```python
from build123d import *

# Parameters (mm, degrees)
F0_W     = 4.2418
F0_H     = 20.1168
F7_DEPTH = 17.78
F1_R     = 2.130855
F2_DEPTH = 7.62
F1_R_2   = 10.202132
F3_DEPTH = 1.27


with BuildPart() as f7:
    # F0 (on Top) → F7 (new body)
    with BuildSketch(Plane.XY):
        Rectangle(F0_W, F0_H)
    extrude(amount=F7_DEPTH)

    # F1 (on offset) → F2 (join)
    with BuildSketch(Plane.XY.offset(17.78)):
        Circle(F1_R)
    extrude(amount=F2_DEPTH)

    # F1 (on offset) → F3 (join)
    with BuildSketch(Plane.XY.offset(17.78)):
        Circle(F1_R_2)
        Circle(F1_R, mode=Mode.SUBTRACT)
    extrude(amount=F3_DEPTH)


solid = f7.part
```
Input: part model. Units: mm. Frame: model coordinates. A direction names the side the tool comes from. Give positions to 0.01 mm unless a question says otherwise; leave off trailing zeros. Loops run counter-clockwise (first coordinate to the right, second up) from the corner with the lowest first, then second, coordinate; pieces in that order, holes last.
1) Section query A-A on x = 0. Return the cut outline in (y, z).
A:
outline: (-10.2, 17.78) - (-10.06, 17.78) - (-10.06, 0) - (10.06, 0) - (10.06, 17.78) - (10.2, 17.78) - (10.2, 19.05) - (2.13, 19.05) - (2.13, 25.4) - (-2.13, 25.4) - (-2.13, 19.05) - (-10.2, 19.05) - close
2) Section query D-D on y = -6. Return the cut outline in (x, z).
A:
outline: (-8.25, 17.78) - (-2.12, 17.78) - (-2.12, 0) - (2.12, 0) - (2.12, 17.78) - (8.25, 17.78) - (8.25, 19.05) - (-8.25, 19.05) - close
3) Reachability of faces 1 (the cylindrical face through (-0.46, -2.08, 22.18)), 2 (the flat face through (2.121, 0, 9)), 3 (the flat face through (-2.121, 0, 9)) from +Z, -Z, +X, -X, +Y, -Y: full face, straight path, thin tool, end or side. Return the list, or none.
A:
face 1: +Z
face 2: -Z, +X, +Y, -Y
face 3: -Z, -X, +Y, -Y
4) Section query C-C on z = 18.5. Return the cut outline in (x, y), and give its area (3 significant figures).
A:
outline: circle Ø20.4 at (0, 0)
area: 327 mm2
5) Line query: L1, parallel to Z at x = 1.75, y = 1.5; L2, parallel to X at y = 7.5, z = 16; L3, parallel to Z at x = -8.75, y = -3. Output: solid intervals per line, ascending.
A:
L1: z = 0 to 19.05
L2: x = -2.12 to 2.12
L3: z = 17.78 to 19.05
6) Contact query for flat-ended pins moving along their axis: pin 1 (1.5 mm diameter, centred on x = -3.5, z = 9, fed in from +Y); pin 2 (2.5 mm diameter, centred on x = 5.5, y = 0, fed in from -Z); pin 3 (5.5 mm diameter, centred on y = 0, z = 11, fed in from -X); pin 4 (6 mm diameter, centred on x = -7, y = -2, fed in from +Z). Output: stop coordinate, or through.
A:
pin 1: passes through
pin 2: stops at z = 17.78
pin 3: stops at x = -2.12
pin 4: stops at z = 19.05
7) Section query B-B on y = -1.25. Return the cut outline in (x, z), and give its area (3 significant figures).
A:
outline: (-10.13, 17.78) - (-2.12, 17.78) - (-2.12, 0) - (2.12, 0) - (2.12, 17.78) - (10.13, 17.78) - (10.13, 19.05) - (1.73, 19.05) - (1.73, 25.4) - (-1.73, 25.4) - (-1.73, 19.05) - (-10.13, 19.05) - close
area: 123 mm2
